Input: part model. Units: mm. Frame: model coordinates. Round coordinates to 2 decimals unless told otherwise and drop trailing zeros. Loops run counter-clockwise (first coordinate to the right, second up) from the corner with the lowest first, then second, coordinate; pieces in that order, holes last. Notation, with made-up numbers: M -31,-10 L 17,-10 A38 cw 17,28 Z; hole C 76,-29.5 d2. An arc over 180 degrees is marked long. Put each result on its own line as item: value. Start each with the question number.
1) Section A-A on x = 20. Output: boundary loops of the cut face in (y, z), plus the area to 3 significant figures.
2) Line query: probe 1 along X at (y, z) = (3.8, -45); probe 2 along Z at (x, y) = (-21, 1.35); probe 3 along Z at (x, y) = (-19.5, 3). Output: solid intervals per line, ascending.
3) Pin query (flat end, axial travel): pin 1 (1.3 mm diameter, centred on x = -4.59, z = -3.12, fed in from +Y). Return the tip coordinate at first contact, or that it passes through.
4) Section B-B on z = 45. Output: boundary loops of the cut face in (x, y), plus the area to 3 significant figures.
5) Section C-C on y = 1.3. Output: boundary loops of the cut face in (x, z).
from build123d import *

# Parameters (mm, degrees)
SKETCH1_W               = 50
SKETCH1_H               = 100
BOSS_EXTRUDE1_DEPTH     = 5
CUT_EXTRUDE1_DEPTH      = 57.124860802
CUT_EXTRUDE1_DEPTH_BACK = 6
SKETCH2_R               = 0.791259191
CUT_EXTRUDE2_DEPTH      = 57.124860802
CUT_EXTRUDE2_DEPTH_BACK = 57.124860802
SKETCH2_3_R             = 0.791259191
CUT_EXTRUDE3_DEPTH      = 57.124860802
CUT_EXTRUDE3_DEPTH_BACK = 57.124860802
SKETCH3_R               = 2.5


with BuildPart() as part:
    # Sketch1 → Boss-Extrude1 (new body)
    with BuildSketch(Plane(origin=(0, 0, 0), x_dir=(1, 0, 0), z_dir=(0, 1, 0))):
        Rectangle(SKETCH1_W, SKETCH1_H)
    extrude(amount=BOSS_EXTRUDE1_DEPTH)

    # Sketch2 → Cut-Extrude1 (cut, two sides: drawn at the far end of the back side and taken through both)
    with BuildSketch(Plane(origin=(0, 5, 0), x_dir=(1, 0, 0), z_dir=(0, 1, 0)).offset(-CUT_EXTRUDE1_DEPTH_BACK)):
        with Locations(Location((-4.591141379, 3.116041861, 0), (0, 0, 90))):
            Circle(SKETCH2_R)
    extrude(amount=CUT_EXTRUDE1_DEPTH + CUT_EXTRUDE1_DEPTH_BACK, mode=Mode.SUBTRACT)

    # Sketch2_3 → Cut-Extrude2 (cut, two sides: drawn at the far end of the back side and taken through both)
    with BuildSketch(Plane(origin=(0, 5, 0), x_dir=(1, 0, 0), z_dir=(0, 1, 0)).offset(-CUT_EXTRUDE2_DEPTH_BACK)):
        with Locations(Location((5.408858621, 3.116041861, 0), (0, 0, 270))):
            Circle(SKETCH2_3_R)
    extrude(amount=CUT_EXTRUDE2_DEPTH + CUT_EXTRUDE2_DEPTH_BACK, mode=Mode.SUBTRACT)

    # Sketch3 → Cut-Extrude3 (cut, two sides: drawn at the far end of the back side and taken through both)
    with BuildSketch(Plane.XZ.offset(-CUT_EXTRUDE3_DEPTH_BACK)):
        with Locations(Location((-20, 45, 0), (0, 0, 270))):
            Circle(SKETCH3_R)
        with Locations(Location((20, 45, 0), (0, 0, 90))):
            Circle(SKETCH3_R)
        with Locations(Location((20, -45, 0), (0, 0, 270))):
            Circle(SKETCH3_R)
        with Locations(Location((-20, -45, 0), (0, 0, 90))):
            Circle(SKETCH3_R)
    extrude(amount=CUT_EXTRUDE3_DEPTH + CUT_EXTRUDE3_DEPTH_BACK, mode=Mode.SUBTRACT)


solid = part.part
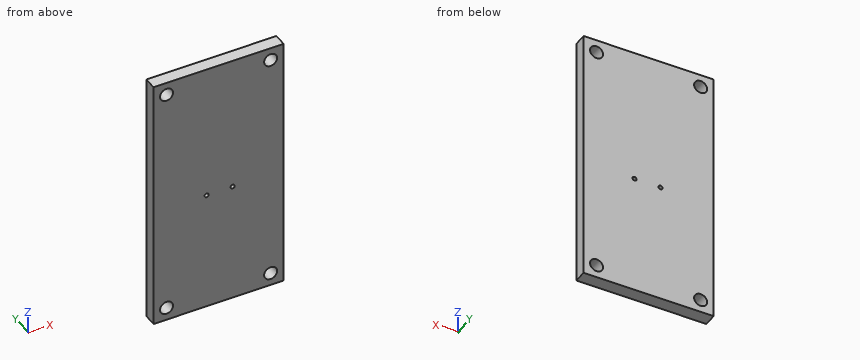
Geometry results:
1. outline: M 0,-50 L 5,-50 L 5,-47.5 L 0,-47.5 Z; M 0,-42.5 L 5,-42.5 L 5,42.5 L 0,42.5 Z; M 0,47.5 L 5,47.5 L 5,50 L 0,50 Z
1. area: 450 mm²
2. probe 1: x = -25 to -22.5, -17.5 to 17.5, 22.5 to 25
2. probe 2: z = -50 to -47.29, -42.71 to 42.71, 47.29 to 50
2. probe 3: z = -50 to -47.45, -42.55 to 42.55, 47.45 to 50
3. pin 1: passes through
4. outline: M -25,0 L -22.5,0 L -22.5,5 L -25,5 Z; M -17.5,0 L 17.5,0 L 17.5,5 L -17.5,5 Z; M 22.5,0 L 25,0 L 25,5 L 22.5,5 Z
4. area: 200 mm²
5. outline: M -25,-50 L 25,-50 L 25,50 L -25,50 Z; hole C -20,-45 d5; hole C -20,45 d5; hole C -4.59,-3.12 d1.58; hole C 5.41,-3.12 d1.58; hole C 20,-45 d5; hole C 20,45 d5
